from build123d import *

# Parameters (mm, degrees)
F0_R     = 2
F1_DEPTH = 6
F2_R     = 3.5
F2_R_2   = 2.75
F3_DEPTH = 1
F4_R     = 4.4
F5_DEPTH = 4
F6_W     = 13
F6_H     = 6
F7_DEPTH = 23
F9_DEPTH = 10


with BuildPart() as f1:
    # F0 (on Front) → F1 (new body)
    with BuildSketch(Plane.XZ):
        with BuildLine():
            Line((0, 3), (32.554146, 0))
            Line((32.554146, 0), (61.188469, 0))
            Line((61.188469, 0), (63.609742, 0))
            ThreePointArc((63.609742, 0), (65.29669, 4.018384), (68.75, 1.359841))
            ThreePointArc((68.75, 1.359841), (68.658544, 0.65653), (68.390258, 0))
            Line((68.390258, 0), (70.811531, 0))
            Line((70.811531, 0), (113, 0))
            Line((113, 0), (115.5, 0))
            ThreePointArc((115.5, 0), (119, 3.5), (122.5, 0))
            Line((122.5, 0), (125, 0))
            Line((125, 0), (125, 1.644468))
            ThreePointArc((125, 1.644468), (124.341818, 4.124108), (122.540554, 5.950927))
            Line((122.540554, 5.950927), (117.372112, 9))
            Line((117.372112, 9), (0, 9))
            Line((0, 9), (0, 3))
        make_face()
        with Locations((46, 4.333029)):
            Circle(F0_R, mode=Mode.SUBTRACT)
        with Locations((89, 4.333029)):
            Circle(F0_R, mode=Mode.SUBTRACT)
        with BuildLine():
            Line((63.609742, 0), (61.188469, 0))
            ThreePointArc((61.188469, 0), (66, -3.640159), (70.811531, 0))
            Line((70.811531, 0), (68.390258, 0))
            ThreePointArc((68.390258, 0), (66, -1.390159), (63.609742, 0))
        make_face()
        with BuildLine():
            ThreePointArc((0, 9), (-3, 6), (0, 3))
            Line((0, 3), (0, 9))
        make_face()
        with BuildLine():
            Line((115.5, 0), (113, 0))
            ThreePointArc((113, 0), (119, -6), (125, 0))
            Line((125, 0), (122.5, 0))
            ThreePointArc((122.5, 0), (119, -3.5), (115.5, 0))
        make_face()
    extrude(amount=F1_DEPTH)

    # F2 (on face) → F3 (join)
    with BuildSketch(Plane(origin=(0, 0, 0), x_dir=(-1, 0, 0), z_dir=(0, 1, 0))):
        with Locations((-66, 1.359841)):
            Circle(F2_R)
        with Locations((-66, 1.359841)):
            Circle(F2_R_2, mode=Mode.SUBTRACT)
    extrude(amount=F3_DEPTH)

    # F4 (on face) → F5 (cut)
    with BuildSketch(Plane.XZ.offset(6)):
        with Locations((119, 0)):
            Circle(F4_R)
    extrude(amount=-F5_DEPTH, mode=Mode.SUBTRACT)

    # F6 (on face) → F7 (join)
    with BuildSketch(Plane(origin=(0, 0, 0), x_dir=(-1, 0, 0), z_dir=(0, 1, 0))):
        with BuildLine():
            Line((0, 9), (0, 3))
            ThreePointArc((0, 3), (3, 6), (0, 9))
        make_face()
        with Locations((-6.5, 6)):
            Rectangle(F6_W, F6_H)
        with BuildLine():
            ThreePointArc((-13, 9), (-16, 6), (-13, 3))
            Line((-13, 3), (-13, 9))
        make_face()
    extrude(amount=F7_DEPTH)

    # F8 (on face) → F9 (cut)
    with BuildSketch(Plane(origin=(0, 23, 0), x_dir=(-1, 0, 0), z_dir=(0, 1, 0))):
        with BuildLine():
            Line((0, 8), (-13, 8))
            ThreePointArc((-13, 8), (-15, 6), (-13, 4))
            Line((-13, 4), (0, 4))
            ThreePointArc((0, 4), (2, 6), (0, 8))
        make_face()
    extrude(amount=-F9_DEPTH, mode=Mode.SUBTRACT)


solid = f1.part
Build history of the part. All positions in model axes, mm. A direction names the side the tool comes from. Round coordinates to 2 decimals unless told otherwise and drop trailing zeros. Write each loop counter-clockwise with the first axis right and the second up, starting at its lowest first coordinate (ties: lowest second). Pieces come first, ordered by that corner, then holes. Notation, with made-up numbers: M 16.5,-10 L 47.5,-10 A22 cw 47.5,18 Z; hole C 62,72.25 d1. An arc over 180 degrees is marked long. Answer in a Markdown table with one row per item.
1. Saw through at A-A (x = 66). List the corners of the cut face in (y, z), and give its area (3 significant figures).
Geometry check:
| item | result |
|---|---|
| outline | M -6,-3.64 L 0,-3.64 L 0,-2.14 L 1,-2.14 L 1,-1.39 L -6,-1.39 Z; M -6,4.11 L 1,4.11 L 1,4.86 L 0,4.86 L 0,9 L -6,9 Z |
| area | 44.3 mm2 |
2. Probe L1, parallel to Z at x = 46, y = -3.8; L2, parallel to Z at x = 66, y = 0.85; L3, parallel to Z at x = 83, y = -3. List the from-to ranges inside material, lowest first. Write a range as [from, to].
Geometry check:
| item | result |
|---|---|
| L1 | [0, 2.33], [6.33, 9] |
| L2 | [-2.14, -1.39], [4.11, 4.86] |
| L3 | [0, 9] |
3. Saw through at D-D (x = 10.5). List the corners of the cut face in (y, z).
Geometry check:
| item | result |
|---|---|
| outline | M -6,2.03 L 0,2.03 L 0,3 L 23,3 L 23,4 L 13,4 L 13,8 L 23,8 L 23,9 L -6,9 Z |
4. Saw through at B-B (x = 46). List the corners of the cut face in (y, z), and give its area (3 significant figures).
Geometry check:
| item | result |
|---|---|
| outline | M -6,0 L 0,0 L 0,2.33 L -6,2.33 Z; M -6,6.33 L 0,6.33 L 0,9 L -6,9 Z |
| area | 30.0 mm2 |
5. Flat gauge pins, fed straight in: P1, Ø5, axis at x = 47.5, z = 0, coming from the +Y side; P2, Ø4.5, axis at x = 89, z = 4.33, coming from the -Y side; P3, Ø1, axis at y = 19.5, z = 3.5, coming from the +X side; P4, Ø1.2, axis at x = 4.5, z = 6.5, coming from the +Y side. Where does each tip first touch, or does it go through?
Geometry check:
| item | result |
|---|---|
| P1 | y = 0 |
| P2 | y = -6 |
| P3 | x = 15.24 |
| P4 | y = 13 |
6. Mould opens along Z. For faces 1 (the face through (47, -3, 0)), 2 (the face through (16, 11, 6)), 3 (the face through (124.36, -2.96, 4.09)), 4 (the face through (7, 13, 6)) say: +Z half, -Z half, draft (parallel to the pull), parting line (faces both ways), or undercut.
Geometry check:
| item | result |
|---|---|
| face 1 | -Z half |
| face 2 | parting line |
| face 3 | +Z half |
| face 4 | undercut |
7. Saw through at C-C (y = 2.5). List the corners of the cut face in (x, z).
Geometry check:
| item | result |
|---|---|
| outline | M 0,3 L 13,3 A3 ccw 13,9 L 0,9 A3 ccw Z |
8. Which spindle directions (+Z, -Z, +X, -X, +Y, -Y) get a long thin tool onto all of the face, cutting with end or side? Do faces 5 (the face through (68.6, 0.5, 3.7)), 6 (the face through (64, 1, -1)), 7 (the face through (92, -3, 0)). Say none if no direction does.
Geometry check:
| item | result |
|---|---|
| face 5 | +Y |
| face 6 | +Z, -Z, +X, +Y |
| face 7 | -Z, +Y, -Y |
